Work out the finished part from the listing and answer in its coordinate system (mm). Face numbers are marked on the shaded views. A direction names the side the tool comes from. Round coordinates to 2 decimals unless told otherwise and drop trailing zeros. Order: outer loops, then holes, each group sorted by start corner. A loop starts at its lowest first (then second) coordinate and runs counter-clockwise, first axis right, second up. Notation, with made-up numbers: (-38.5, 72) -> (-31.5, 72) arc R28 ccw to (-31.5, 96) -> close; hole circle Ø11 at (-13.75, 17). An arc over 180 degrees is marked (long way). Use a Markdown table: item, result. Add a question column.
Item 1: A cutting plane is placed at C-C, the plane x = -16. Determine the outline of the cut face in (y, z).
Item 2: A cutting plane is placed at A-A, the plane z = 11. Determine the outline of the cut face in (x, y), plus the area to 3 significant figures.
Item 3: A cutting plane is placed at D-D, the plane z = 19. Determine the outline of the cut face in (x, y).
Item 4: For a pull along X with two mould halves and no side action, classify the marked faces 3, 4 and 5 as +X half, -X half, draft (parallel to the pull), parting line (faces both ways), or undercut.
Item 5: A cutting plane is placed at B-B, the plane x = 11.5. Determine the outline of the cut face in (y, z).
Item 6: A tool of negligible diameter and unlimited length cuts with its end or side. For the marked faces 1 and 2, from which of +Z, -Z, +X, -X, +Y, -Y can it reach the whole face along a straight path? Write none if from no direction.
Item 7: Find the intervals of material crossed by L1, parallel to X at y = 8.75, z = 0.5; L2, parallel to Z at x = 17, y = 9.75; L3, parallel to Y at x = 11.5, z = -31.35, in increasing order. Write a range as [from, to].
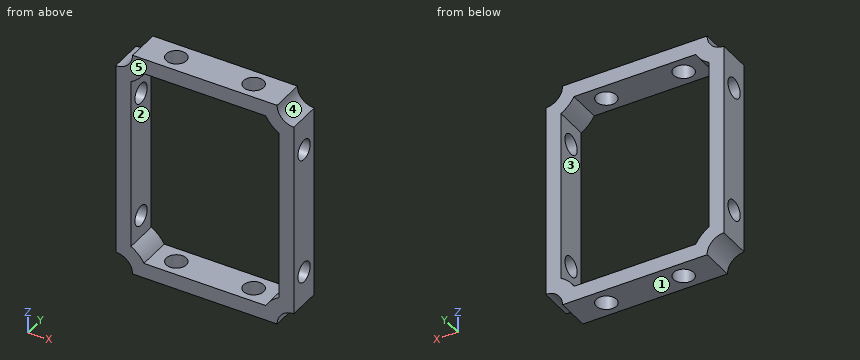
from build123d import *

# Parameters (mm, degrees)
BOSS_EXTRUDE1_DEPTH = 10
SKETCH2_R           = 3
CUT_EXTRUDE1_DEPTH  = 64.757352517
SKETCH3_R           = 3
CUT_EXTRUDE2_DEPTH  = 74.663084377


with BuildPart() as part:
    # Sketch1 → Boss-Extrude1 (new body)
    with BuildSketch(Plane(origin=(0, 0, 0), x_dir=(1, 0, 0), z_dir=(0, 1, 0))):
        with BuildLine():
            Line((-21.5, 34), (21.5, 34))
            ThreePointArc((21.5, 34), (22.964466094, 30.464466094), (26.5, 29))
            Line((26.5, 29), (26.5, -29))
            ThreePointArc((26.5, -29), (22.964466094, -30.464466094), (21.5, -34))
            Line((21.5, -34), (-21.5, -34))
            ThreePointArc((-21.5, -34), (-22.964466094, -30.464466094), (-26.5, -29))
            Line((-26.5, -29), (-26.5, 29))
            ThreePointArc((-26.5, 29), (-22.964466094, 30.464466094), (-21.5, 34))
        make_face()
        with BuildLine():
            Line((-22, 25.633399735), (-22, -25.633399735))
            ThreePointArc((-22, -25.633399735), (-19.782485579, -27.282485579), (-18.133399735, -29.5))
            Line((-18.133399735, -29.5), (18.133399735, -29.5))
            ThreePointArc((18.133399735, -29.5), (19.782485579, -27.282485579), (22, -25.633399735))
            Line((22, -25.633399735), (22, 25.633399735))
            ThreePointArc((22, 25.633399735), (19.782485579, 27.282485579), (18.133399735, 29.5))
            Line((18.133399735, 29.5), (-18.133399735, 29.5))
            ThreePointArc((-18.133399735, 29.5), (-19.782485579, 27.282485579), (-22, 25.633399735))
        make_face(mode=Mode.SUBTRACT)
    extrude(amount=BOSS_EXTRUDE1_DEPTH)

    # Sketch2 → Cut-Extrude1 (cut, through all)
    with BuildSketch(Plane(origin=(26.5, 0, 0), x_dir=(0, 0, -1), z_dir=(1, 0, 0))):
        with Locations((-19, 5)):
            Circle(SKETCH2_R)
        with Locations((19, 5)):
            Circle(SKETCH2_R)
    extrude(amount=-CUT_EXTRUDE1_DEPTH, mode=Mode.SUBTRACT)

    # Sketch3 → Cut-Extrude2 (cut, through all)
    with BuildSketch(Plane.XY.offset(34)):
        with Locations((11.5, 5)):
            Circle(SKETCH3_R)
        with Locations((-11.5, 5)):
            Circle(SKETCH3_R)
    extrude(amount=-CUT_EXTRUDE2_DEPTH, mode=Mode.SUBTRACT)


solid = part.part
Reported:
| question | item | result |
|---|---|---|
| 1 | outline | (0, -34) -> (10, -34) -> (10, -29.5) -> (0, -29.5) -> close; (0, 29.5) -> (10, 29.5) -> (10, 34) -> (0, 34) -> close |
| 2 | outline | (-26.5, 0) -> (-22, 0) -> (-22, 10) -> (-26.5, 10) -> close; (22, 0) -> (26.5, 0) -> (26.5, 10) -> (22, 10) -> close |
| 2 | area | 90.0 mm² |
| 3 | outline | (-26.5, 0) -> (-22, 0) -> (-22, 2) -> (-26.5, 2) -> close; (-26.5, 8) -> (-22, 8) -> (-22, 10) -> (-26.5, 10) -> close; (22, 0) -> (26.5, 0) -> (26.5, 2) -> (22, 2) -> close; (22, 8) -> (26.5, 8) -> (26.5, 10) -> (22, 10) -> close |
| 4 | face 3 | undercut |
| 4 | face 4 | +X half |
| 4 | face 5 | draft |
| 5 | outline | (0, -34) -> (2, -34) -> (2, -29.5) -> (0, -29.5) -> close; (0, 29.5) -> (2, 29.5) -> (2, 34) -> (0, 34) -> close; (8, -34) -> (10, -34) -> (10, -29.5) -> (8, -29.5) -> close; (8, 29.5) -> (10, 29.5) -> (10, 34) -> (8, 34) -> close |
| 6 | face 1 | -Z, +X, -X, +Y, -Y |
| 6 | face 2 | +Y, -Y |
| 7 | L1 | [-26.5, -22], [22, 26.5] |
| 7 | L2 | [-34, -29.5], [29.5, 34] |
| 7 | L3 | [0, 2], [8, 10] |
